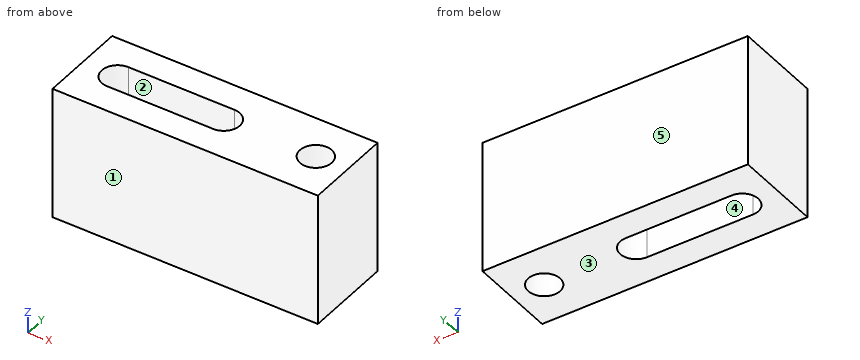
```python
from build123d import *

# Parameters (mm, degrees)
SKETCH1_W           = 1500
SKETCH1_H           = 750
BOSS_EXTRUDE1_DEPTH = 500
SKETCH2_R           = 90
CUT_EXTRUDE1_DEPTH  = 1173.603939956


with BuildPart() as part:
    # Sketch1 → Boss-Extrude1 (new body)
    with BuildSketch(Plane(origin=(0, 0, 0), x_dir=(1, 0, 0), z_dir=(0, 1, 0))):
        Rectangle(SKETCH1_W, SKETCH1_H)
    extrude(amount=BOSS_EXTRUDE1_DEPTH)

    # Sketch2 → Cut-Extrude1 (cut, through all)
    with BuildSketch(Plane.XY.offset(375)):
        with Locations((570, 250)):
            Circle(SKETCH2_R)
        with BuildLine():
            Line((-550, 340), (50, 340))
            ThreePointArc((50, 340), (140, 250), (50, 160))
            Line((50, 160), (-550, 160))
            ThreePointArc((-550, 160), (-640, 250), (-550, 340))
        make_face()
    extrude(amount=-CUT_EXTRUDE1_DEPTH, mode=Mode.SUBTRACT)


solid = part.part
```
Geometry: final body of the model. Coordinates: model frame, mm. Face numbers are marked on the shaded views. A direction names the side the tool comes from. Give positions to 0.01 mm unless a question says otherwise; leave off trailing zeros. Write each loop counter-clockwise with the first axis right and the second up, starting at its lowest first coordinate (ties: lowest second). Pieces come first, ordered by that corner, then holes.
1. Reachability of the marked faces 4 and 5 from +Z, -Z, +X, -X, +Y, -Y: full face, straight path, thin tool, end or side. Return the list, or none.
2. Section query B-B, the plane y = 181. Return loops of the section in (x, z), then the cut area to 3 significant figures.
3. Section query A-A, the plane x = 570. Return loops of the section in (y, z), then the cut area to 3 significant figures.
4. Draft query along Y for the marked faces 1, 2 and 3. Return one class per face: released by +Y, released by -Y, zero draft, split by the parting line, or undercut.
5. Line query: probe 1 along Y at (x, z) = (570, -30); probe 2 along X at (y, z) = (185, 171); probe 3 along Y at (x, z) = (605.5, -74.5). Output: solid intervals per line, ascending.
6. Section query C-C, the plane z = -37.5. Return loops of the section in (x, y), then the cut area to 3 significant figures.
7. Section query D-D, the plane y = 317. Return loops of the section in (x, z).
Computed:
1. face 4: +Z, -Z
1. face 5: +Z, -Z, +X, -X, +Y
2. outline: (-750, -375) - (-607.78, -375) - (-607.78, 375) - (-750, 375) - close; (107.78, -375) - (512.22, -375) - (512.22, 375) - (107.78, 375) - close; (627.78, -375) - (750, -375) - (750, 375) - (627.78, 375) - close
2. area: 502,000 mm2
3. outline: (0, -375) - (160, -375) - (160, 375) - (0, 375) - close; (340, -375) - (500, -375) - (500, 375) - (340, 375) - close
3. area: 240,000 mm2
4. face 1: released by -Y
4. face 2: undercut
4. face 3: zero draft
5. probe 1: y = 0 to 160, 340 to 500
5. probe 2: x = -750 to -612.25, 112.25 to 507.75, 632.25 to 750
5. probe 3: y = 0 to 167.3, 332.7 to 500
6. outline: (-750, 0) - (750, 0) - (750, 500) - (-750, 500) - close; hole (-550, 160) - (50, 160) arc R90 ccw to (50, 340) - (-550, 340) arc R90 ccw to start; hole circle Ø180 at (570, 250)
6. area: 591,000 mm2
7. outline: (-750, -375) - (-610.09, -375) - (-610.09, 375) - (-750, 375) - close; (110.09, -375) - (509.91, -375) - (509.91, 375) - (110.09, 375) - close; (630.09, -375) - (750, -375) - (750, 375) - (630.09, 375) - close
